Check sheet for the modelled part. Datum: model origin and axes. Units: mm. Give positions to 0.01 mm unless a question says otherwise; leave off trailing zeros. Order: outer loops, then holes, each group sorted by start corner. A loop starts at its lowest first (then second) coordinate and runs counter-clockwise, first axis right, second up.
from build123d import *

# Parameters (mm, degrees)
F0_R     = 27
F0_R_2   = 11.4
F1_DEPTH = 1
F3_DEPTH = 1
F4_SIZE  = 0.5


with BuildPart() as f1:
    # F0 (on Top) → F1 (new body)
    with BuildSketch(Plane.XY):
        Circle(F0_R)
        Circle(F0_R_2, mode=Mode.SUBTRACT)
    extrude(amount=F1_DEPTH)

    # F2 (on face) → F3 (cut, through all)
    with BuildSketch(Plane.XY.offset(1)):
        with BuildLine():
            ThreePointArc((0.1, 26.999815), (0, 27), (-0.1, 26.999815))
            Line((-0.1, 26.999815), (-0.1, 11.399561))
            Line((-0.1, 11.399561), (0.1, 11.399561))
            Line((0.1, 11.399561), (0.1, 26.999815))
        make_face()
    extrude(amount=-F3_DEPTH, mode=Mode.SUBTRACT)

    # F4
    f4_edges = [f1.edges().sort_by_distance(p)[0] for p in [
        (-19.056495, -19.127206, 0),
        (-8.025584, -8.096295, 0),
    ]]
    chamfer(f4_edges, length=F4_SIZE)


solid = f1.part
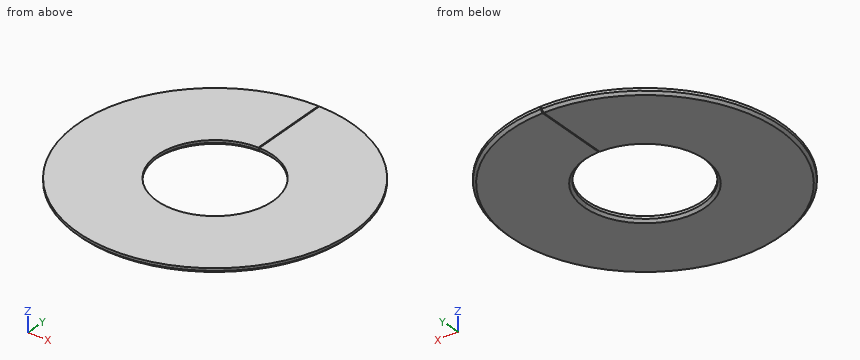
1) Material ranges on L1, parallel to X at y = 0, z = 0.8; L2, parallel to Y at x = 0, z = 0.6; L3, parallel to Y at x = 5.5, z = 0.55, recorded low to high.
Recorded:
L1: x = -27 to -11.4, 11.4 to 27
L2: y = -27 to -11.4
L3: y = -26.43 to -9.99, 9.99 to 26.43
2) Section check A-A, the plane z = 0.7. Record the cut outline in (x, y).
Recorded:
outline: (-0.1, 11.4) - (-0.1, 27) arc R27 ccw (long way) to (0.1, 27) - (0.1, 11.4) arc R11.4 cw (long way) to start
3) Depth check by flat-ended pin: pin 1 Ø18 at (x, y) = (0, 0) entering from -Z. Enter the tip coordinate at first touch or a pass-through.
Recorded:
pin 1: passes through
